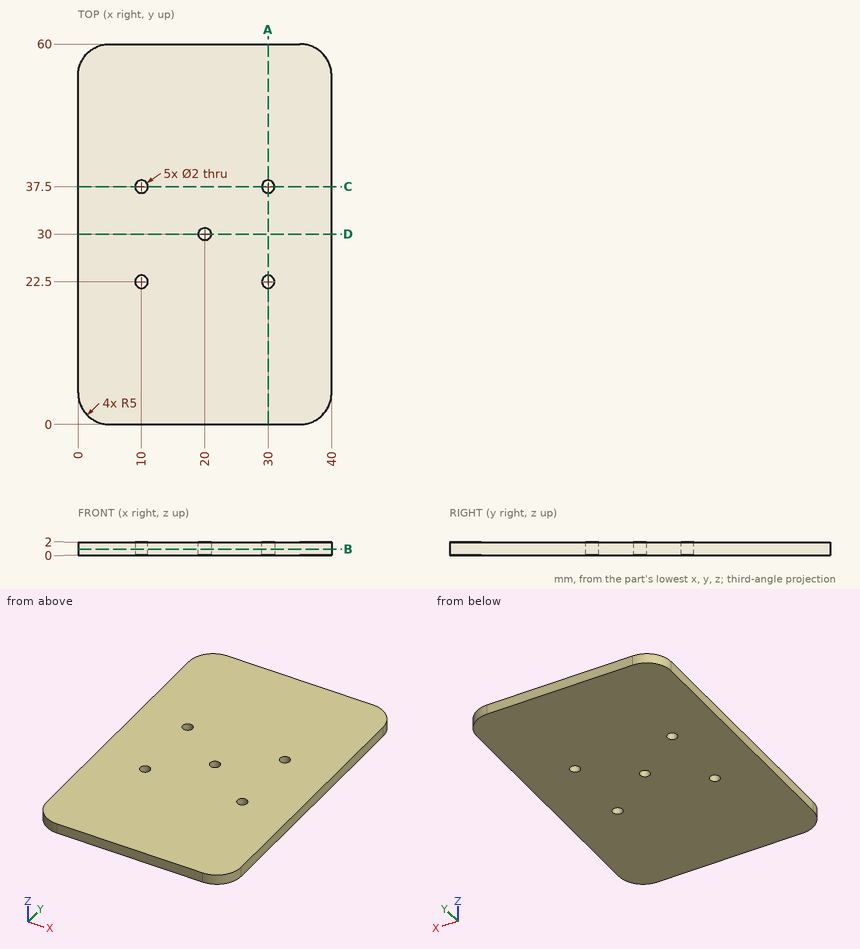
Here's the drawing with two shaded views (mm, measured from the low corner). I have some questions. Give positions to 0.01 mm unless a question says otherwise; leave off trailing zeros. Write each loop counter-clockwise with the first axis right and the second up, starting at its lowest first coordinate (ties: lowest second). Pieces come first, ordered by that corner, then holes. Notation, with made-up numbers: (-24.75, -17.5) -> (7.25, -17.5) arc R24 cw to (7.25, 6.5) -> close; hole circle Ø5 at (40.25, -19.5). An arc over 180 degrees is marked (long way). Use one line per item in the form item = value.
1) Suppose I cut it at A-A (x = 30). Please give me the cut outline in (y, z), and give its area (3 significant figures).
Verdict:
outline = (0, 0) -> (21.5, 0) -> (21.5, 2) -> (0, 2) -> close; (23.5, 0) -> (36.5, 0) -> (36.5, 2) -> (23.5, 2) -> close; (38.5, 0) -> (60, 0) -> (60, 2) -> (38.5, 2) -> close
area = 112 mm2
2) Suppose I cut it at B-B (z = 0.95). Please give me the cut outline in (x, y).
Verdict:
outline = (0, 5) arc R5 ccw to (5, 0) -> (35, 0) arc R5 ccw to (40, 5) -> (40, 55) arc R5 ccw to (35, 60) -> (5, 60) arc R5 ccw to (0, 55) -> close; hole circle Ø2 at (10, 22.5); hole circle Ø2 at (10, 37.5); hole circle Ø2 at (20, 30); hole circle Ø2 at (30, 22.5); hole circle Ø2 at (30, 37.5)
3) I'm going to push a flat-ended pin straight in: pin 1 (1.8 mm diameter, centred on x = 30, y = 37.5, fed in from -Z). Where does the tip first touch, or does it pass through?
Verdict:
pin_1 = through
4) If I drill on L1, parallel to Y at x = 30, z = 0.7; L2, parallel to Y at x = 20.5, z = 1.05; L3, parallel to X at y = 3.5, z = 0.85, over which ranges is the centre line in solid material (lowest first)? Write a range as [from, to].
Verdict:
L1 = [0, 21.5], [23.5, 36.5], [38.5, 60]
L2 = [0, 29.13], [30.87, 60]
L3 = [0.23, 39.77]
5) Suppose I cut it at D-D (y = 30). Please give me the cut outline in (x, z).
Verdict:
outline = (0, 0) -> (19, 0) -> (19, 2) -> (0, 2) -> close; (21, 0) -> (40, 0) -> (40, 2) -> (21, 2) -> close
6) Suppose I cut it at C-C (y = 37.5). Please give me the cut outline in (x, z).
Verdict:
outline = (0, 0) -> (9, 0) -> (9, 2) -> (0, 2) -> close; (11, 0) -> (29, 0) -> (29, 2) -> (11, 2) -> close; (31, 0) -> (40, 0) -> (40, 2) -> (31, 2) -> close
